```python
from build123d import *

# Parameters (mm, degrees)
F0_R     = 8.89
F1_DEPTH = 12.7
F0_W     = 34.590188
F0_H     = 111.76
F2_DEPTH = 0.762
F3_R     = 5.08


with BuildPart() as f1:
    # F0 (on Top) → F1 (new body)
    with BuildSketch(Plane.XY):
        Polygon((80.518, -57.15), (80.518, 57.15), (-80.518, 57.15), (-80.518, 55.88), (-80.518, -55.88), (-80.518, -57.15), align=None)
        with Locations((-67.818, -44.45)):
            Circle(F0_R, mode=Mode.SUBTRACT)
        with Locations((-45.212, -44.45)):
            Circle(F0_R, mode=Mode.SUBTRACT)
        with Locations((-22.606, -44.45)):
            Circle(F0_R, mode=Mode.SUBTRACT)
        with Locations((-67.818, -22.225)):
            Circle(F0_R, mode=Mode.SUBTRACT)
        with Locations((-45.212, -22.225)):
            Circle(F0_R, mode=Mode.SUBTRACT)
        with Locations((-22.606, -22.225)):
            Circle(F0_R, mode=Mode.SUBTRACT)
        with Locations((0, -44.45)):
            Circle(F0_R, mode=Mode.SUBTRACT)
        with Locations((22.606, -44.45)):
            Circle(F0_R, mode=Mode.SUBTRACT)
        with Locations((45.212, -44.45)):
            Circle(F0_R, mode=Mode.SUBTRACT)
        with Locations((67.818, -44.45)):
            Circle(F0_R, mode=Mode.SUBTRACT)
        with Locations((0, -22.225)):
            Circle(F0_R, mode=Mode.SUBTRACT)
        with Locations((22.606, -22.225)):
            Circle(F0_R, mode=Mode.SUBTRACT)
        with Locations((45.212, -22.225)):
            Circle(F0_R, mode=Mode.SUBTRACT)
        with Locations((67.818, -22.225)):
            Circle(F0_R, mode=Mode.SUBTRACT)
        with Locations((-67.818, 0)):
            Circle(F0_R, mode=Mode.SUBTRACT)
        with Locations((-67.818, 22.225)):
            Circle(F0_R, mode=Mode.SUBTRACT)
        with Locations((-45.212, 0)):
            Circle(F0_R, mode=Mode.SUBTRACT)
        with Locations((-22.606, 0)):
            Circle(F0_R, mode=Mode.SUBTRACT)
        with Locations((-45.212, 22.225)):
            Circle(F0_R, mode=Mode.SUBTRACT)
        with Locations((-22.606, 22.225)):
            Circle(F0_R, mode=Mode.SUBTRACT)
        with Locations((-67.818, 44.45)):
            Circle(F0_R, mode=Mode.SUBTRACT)
        with Locations((-45.212, 44.45)):
            Circle(F0_R, mode=Mode.SUBTRACT)
        with Locations((-22.606, 44.45)):
            Circle(F0_R, mode=Mode.SUBTRACT)
        Circle(F0_R, mode=Mode.SUBTRACT)
        with Locations((22.606, 0)):
            Circle(F0_R, mode=Mode.SUBTRACT)
        with Locations((0, 22.225)):
            Circle(F0_R, mode=Mode.SUBTRACT)
        with Locations((22.606, 22.225)):
            Circle(F0_R, mode=Mode.SUBTRACT)
        with Locations((45.212, 0)):
            Circle(F0_R, mode=Mode.SUBTRACT)
        with Locations((67.818, 0)):
            Circle(F0_R, mode=Mode.SUBTRACT)
        with Locations((45.212, 22.225)):
            Circle(F0_R, mode=Mode.SUBTRACT)
        with Locations((67.818, 22.225)):
            Circle(F0_R, mode=Mode.SUBTRACT)
        with Locations((0, 44.45)):
            Circle(F0_R, mode=Mode.SUBTRACT)
        with Locations((22.606, 44.45)):
            Circle(F0_R, mode=Mode.SUBTRACT)
        with Locations((45.212, 44.45)):
            Circle(F0_R, mode=Mode.SUBTRACT)
        with Locations((67.818, 44.45)):
            Circle(F0_R, mode=Mode.SUBTRACT)
        Polygon((-80.518, 55.88), (-80.518, 57.15), (-116.378188, 57.15), (-116.378188, -57.15), (-80.518, -57.15), (-80.518, -55.88), (-115.108188, -55.88), (-115.108188, 55.88), align=None)
    extrude(amount=F1_DEPTH)

    # F0 (on Top) → F2 (join)
    with BuildSketch(Plane.XY):
        with Locations((-67.818, 44.45)):
            Circle(F0_R)
        with Locations((-45.212, 44.45)):
            Circle(F0_R)
        with Locations((-22.606, 44.45)):
            Circle(F0_R)
        with Locations((0, 44.45)):
            Circle(F0_R)
        with Locations((22.606, 44.45)):
            Circle(F0_R)
        with Locations((45.212, 44.45)):
            Circle(F0_R)
        with Locations((67.818, 44.45)):
            Circle(F0_R)
        with Locations((67.818, 22.225)):
            Circle(F0_R)
        with Locations((45.212, 22.225)):
            Circle(F0_R)
        with Locations((22.606, 22.225)):
            Circle(F0_R)
        with Locations((0, 22.225)):
            Circle(F0_R)
        with Locations((-22.606, 22.225)):
            Circle(F0_R)
        with Locations((-45.212, 22.225)):
            Circle(F0_R)
        with Locations((-67.818, 22.225)):
            Circle(F0_R)
        with Locations((-67.818, 0)):
            Circle(F0_R)
        with Locations((-45.212, 0)):
            Circle(F0_R)
        with Locations((-22.606, 0)):
            Circle(F0_R)
        Circle(F0_R)
        with Locations((22.606, 0)):
            Circle(F0_R)
        with Locations((45.212, 0)):
            Circle(F0_R)
        with Locations((67.818, 0)):
            Circle(F0_R)
        with Locations((67.818, -22.225)):
            Circle(F0_R)
        with Locations((45.212, -22.225)):
            Circle(F0_R)
        with Locations((22.606, -22.225)):
            Circle(F0_R)
        with Locations((0, -22.225)):
            Circle(F0_R)
        with Locations((-22.606, -22.225)):
            Circle(F0_R)
        with Locations((-45.212, -22.225)):
            Circle(F0_R)
        with Locations((-67.818, -22.225)):
            Circle(F0_R)
        with Locations((-67.818, -44.45)):
            Circle(F0_R)
        with Locations((-45.212, -44.45)):
            Circle(F0_R)
        with Locations((-22.606, -44.45)):
            Circle(F0_R)
        with Locations((0, -44.45)):
            Circle(F0_R)
        with Locations((22.606, -44.45)):
            Circle(F0_R)
        with Locations((45.212, -44.45)):
            Circle(F0_R)
        with Locations((67.818, -44.45)):
            Circle(F0_R)
        with Locations((-97.813094, 0)):
            Rectangle(F0_W, F0_H)
    extrude(amount=F2_DEPTH)

    # F3
    f3_edges = [f1.edges().sort_by_distance(p)[0] for p in [
        (80.518, 57.15, 6.35),
        (80.518, -57.15, 6.35),
        (-80.518, -55.88, 6.731),
        (-80.518, 55.88, 6.731),
        (-115.108188, 55.88, 6.731),
        (-115.108188, -55.88, 6.731),
        (-116.378188, -57.15, 6.35),
        (-116.378188, 57.15, 6.35),
    ]]
    fillet(f3_edges, radius=F3_R)


solid = f1.part
```
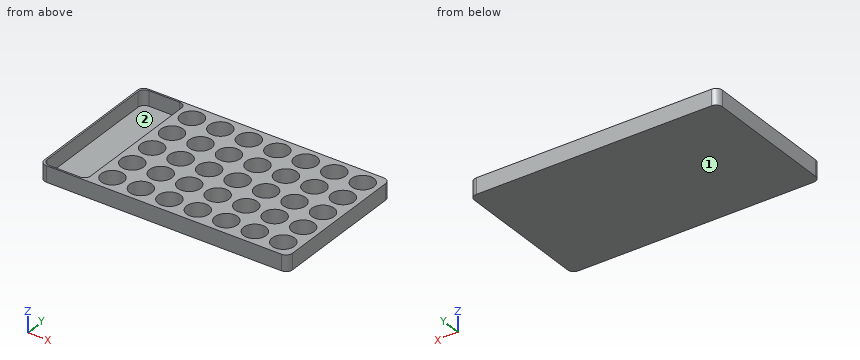
Build history of the part. All positions in model axes, mm. Face numbers are marked on the shaded views. Coordinates: 2 decimals unless noted, no trailing zeros. Order: outer loops, then holes, each group sorted by start corner. A loop starts at its lowest first (then second) coordinate and runs counter-clockwise, first axis right, second up.
Item 1: Saw through at B-B on x = -43.5. List the corners of the cut face in (y, z), then the cut area to 3 significant figures.
Filled in:
outline: (-57.15, 0) - (57.15, 0) - (57.15, 12.7) - (53.17, 12.7) - (53.17, 0.76) - (35.73, 0.76) - (35.73, 12.7) - (30.95, 12.7) - (30.95, 0.76) - (13.5, 0.76) - (13.5, 12.7) - (8.72, 12.7) - (8.72, 0.76) - (-8.72, 0.76) - (-8.72, 12.7) - (-13.5, 12.7) - (-13.5, 0.76) - (-30.95, 0.76) - (-30.95, 12.7) - (-35.73, 12.7) - (-35.73, 0.76) - (-53.17, 0.76) - (-53.17, 12.7) - (-57.15, 12.7) - close
area: 410 mm2
Item 2: Saw through at C-C on z = 5.75. State how many separate pieces and enclosed holes the cut face has, then the cut area to 3 significant figures.
Filled in:
separate pieces: 1
enclosed holes: 36
area: 9,950 mm2
Item 3: Saw through at A-A on x = -103.5. List the corners of the cut face in (y, z), then the cut area to 3 significant figures.
Filled in:
outline: (-57.15, 0) - (57.15, 0) - (57.15, 12.7) - (55.88, 12.7) - (55.88, 0.76) - (-55.88, 0.76) - (-55.88, 12.7) - (-57.15, 12.7) - close
area: 117 mm2
Item 4: Drill centre lines: L1, parallel to Y at x = -45, z = 7.75; L2, parallel to Y at x = -104.5, z = 9; L3, parallel to Y at x = -5.5, z = 12. Where is each one in solid material? Low to high.
Filled in:
L1: y = -57.15 to -53.34, -35.56 to -31.11, -13.34 to -8.89, 8.89 to 13.34, 31.11 to 35.56, 53.34 to 57.15
L2: y = -57.15 to -55.88, 55.88 to 57.15
L3: y = -57.15 to -51.43, -37.47 to -29.21, -15.24 to -6.98, 6.98 to 15.24, 29.21 to 37.47, 51.43 to 57.15
Item 5: Saw through at D-D on x = 0. List the corners of the cut face in (y, z) (3 decimals), then the cut area to 3 significant figures.
Filled in:
outline: (-57.15, 0) - (57.15, 0) - (57.15, 12.7) - (53.34, 12.7) - (53.34, 0.762) - (35.56, 0.762) - (35.56, 12.7) - (31.115, 12.7) - (31.115, 0.762) - (13.335, 0.762) - (13.335, 12.7) - (8.89, 12.7) - (8.89, 0.762) - (-8.89, 0.762) - (-8.89, 12.7) - (-13.335, 12.7) - (-13.335, 0.762) - (-31.115, 0.762) - (-31.115, 12.7) - (-35.56, 12.7) - (-35.56, 0.762) - (-53.34, 0.762) - (-53.34, 12.7) - (-57.15, 12.7) - close
area: 390 mm2
Item 6: Mould opens along X. For the marked faces 1 and 2 say: released by +X, released by -X, zero draft, split by the parting line, or undercut.
Filled in:
face 1: zero draft
face 2: undercut
Item 7: Drop a flat-ended pin along its axis: pin 1 Ø5.5 at (x, y) = (-47.5, 40.5) entering from +Z. Give the stop position or say it passes through.
Filled in:
pin 1: stops at z = 0.76
